from build123d import *

# Parameters (mm, degrees)
SKETCH1_W           = 19.05
SKETCH1_H           = 107.95
BOSS_EXTRUDE1_DEPTH = 3.175
SKETCH2_W           = 12.7
SKETCH2_H           = 6.35
CUT_EXTRUDE1_DEPTH  = 7.35


with BuildPart() as part:
    # Sketch1 → Boss-Extrude1 (new body, symmetric)
    with BuildSketch(Plane(origin=(0, 0, 0), x_dir=(0, 0, -1), z_dir=(1, 0, 0))):
        Rectangle(SKETCH1_W, SKETCH1_H)
    extrude(amount=BOSS_EXTRUDE1_DEPTH, both=True)

    # Sketch2 → Cut-Extrude1 (cut, through all)
    with BuildSketch(Plane(origin=(3.175, 0, 0), x_dir=(0, 0, -1), z_dir=(1, 0, 0))):
        with Locations((-3.175, 50.8)):
            Rectangle(SKETCH2_W, SKETCH2_H)
        with Locations((-3.175, 17.4625)):
            Rectangle(SKETCH2_W, SKETCH2_H)
    extrude(amount=-CUT_EXTRUDE1_DEPTH, mode=Mode.SUBTRACT)


solid = part.part
Design review of the part built by this model. Coordinates are the model's own, in mm. A direction names the side the tool comes from. Coordinates: 2 decimals unless noted, no trailing zeros. Order: outer loops, then holes, each group sorted by start corner. A loop starts at its lowest first (then second) coordinate and runs counter-clockwise, first axis right, second up. Notation, with made-up numbers: (48, 51) -> (70, 51) arc R22 cw to (70, 68) -> close; hole circle Ø7 at (15.25, 58.25). An arc over 180 degrees is marked (long way). Use one line per item in the form item = value. Start each with the question number.
(1) The part is to be moulded in two halves that separate along Y. For faces 1 (the flat face through (0, 14.287, 3)), 2 (the flat face through (0, -53.975, 0)), 3 (the flat face through (0, -1, -9.525)), 4 (the flat face through (0, 47.625, 3)), say which applies: +Y half, -Y half, draft (parallel to the pull), parting line (faces both ways), or undercut.
(2) Insertion check: pin 1 (1.9 mm diameter, centred on x = 0.5, y = 17.5, fed in from +Z) (3 decimals); pin 2 (1.5 mm diameter, centred on x = -1.5, z = -1.5, fed in from +Y) (3 decimals). Each pin has a flat end and moves straight along its axis. Give the tip position at first contact, or say it passes through.
(3) Add section B-B on x = 2. State the section outline as (y, z) points (1 decimal), plus the area to 3 significant figures.
(4) Add section A-A on z = 1. State the section outline as (x, y) points (1 decimal), plus the area to 3 significant figures.
(5) For faces 5 (the flat face through (0, 51, -3.175)), 6 (the flat face through (0, 20.638, 3)), 7 (the flat face through (0, -20, 9.525)), list the 3-axis set-ups (+Z, -Z, +X, -X, +Y, -Y) from which the entire face can be reached by the end or side of a thin tool; tool diameter is ignored.
(6) For probe 1 along Y at (x, z) = (2.5, 6.5) (1 decimal), list the stretches that pass through material, from the lowest coordinate up.
Answer block:
q1.face_1 = undercut
q1.face_2 = -Y half
q1.face_3 = draft
q1.face_4 = +Y half
q2.pin_1 = -3.175
q2.pin_2 = 47.625
q3.outline = (-54, -9.5) -> (54, -9.5) -> (54, -3.2) -> (47.6, -3.2) -> (47.6, 9.5) -> (20.6, 9.5) -> (20.6, -3.2) -> (14.3, -3.2) -> (14.3, 9.5) -> (-54, 9.5) -> close
q3.area = 1,900 mm²
q4.outline = (-3.2, -54) -> (3.2, -54) -> (3.2, 14.3) -> (-3.2, 14.3) -> close; (-3.2, 20.6) -> (3.2, 20.6) -> (3.2, 47.6) -> (-3.2, 47.6) -> close
q4.area = 605 mm²
q5.face_5 = +Z, +X, -X, +Y
q5.face_6 = +Z, +X, -X
q5.face_7 = +Z, +X, -X, +Y, -Y
q6.probe_1 = -54 to 14.3, 20.6 to 47.6
